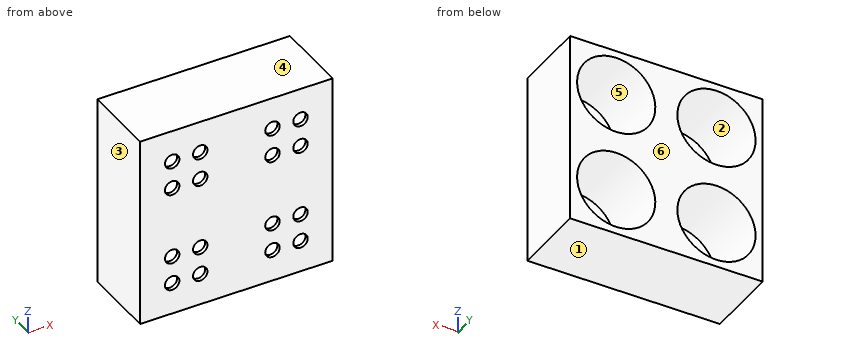
```python
from build123d import *

# Parameters (mm, degrees)
SKETCH1_W           = 96
SKETCH1_H           = 96
SKETCH1_R           = 19.5
BOSS_EXTRUDE1_DEPTH = 35
SKETCH2_W           = 96
SKETCH2_H           = 96
BOSS_EXTRUDE2_DEPTH = 2
SKETCH3_R           = 3.6
CUT_EXTRUDE1_DEPTH  = 110.009173926


with BuildPart() as part:
    # Sketch1 → Boss-Extrude1 (new body)
    with BuildSketch(Plane(origin=(0, 0, 0), x_dir=(1, 0, 0), z_dir=(0, 1, 0))):
        with Locations((25, 25)):
            Rectangle(SKETCH1_W, SKETCH1_H)
        with Locations(Location((0, 0, 0), (0, 0, 270))):
            Circle(SKETCH1_R, mode=Mode.SUBTRACT)
        with Locations(Location((50, 0, 0), (0, 0, 270))):
            Circle(SKETCH1_R, mode=Mode.SUBTRACT)
        with Locations(Location((50, 50, 0), (0, 0, 270))):
            Circle(SKETCH1_R, mode=Mode.SUBTRACT)
        with Locations(Location((0, 50, 0), (0, 0, 270))):
            Circle(SKETCH1_R, mode=Mode.SUBTRACT)
    extrude(amount=BOSS_EXTRUDE1_DEPTH)

    # Sketch2 → Boss-Extrude2 (add)
    with BuildSketch(Plane.XZ):
        with Locations((25, -25)):
            Rectangle(SKETCH2_W, SKETCH2_H)
    extrude(amount=BOSS_EXTRUDE2_DEPTH)

    # Sketch3 → Cut-Extrude1 (cut, through all)
    with BuildSketch(Plane(origin=(0, 0, 0), x_dir=(1, 0, 0), z_dir=(0, 1, 0))):
        with Locations(Location((57, 43, 0), (0, 0, 270))):
            Circle(SKETCH3_R)
        with Locations(Location((57, 57, 0), (0, 0, 90))):
            Circle(SKETCH3_R)
        with Locations(Location((43, 43, 0), (0, 0, 90))):
            Circle(SKETCH3_R)
        with Locations(Location((43, 57, 0), (0, 0, 270))):
            Circle(SKETCH3_R)
        with Locations(Location((57, 7, 0), (0, 0, 270))):
            Circle(SKETCH3_R)
        with Locations(Location((43, 7, 0), (0, 0, 90))):
            Circle(SKETCH3_R)
        with Locations(Location((43, -7, 0), (0, 0, 270))):
            Circle(SKETCH3_R)
        with Locations(Location((57, -7, 0), (0, 0, 90))):
            Circle(SKETCH3_R)
        with Locations(Location((7, 7, 0), (0, 0, 270))):
            Circle(SKETCH3_R)
        with Locations(Location((7, -7, 0), (0, 0, 90))):
            Circle(SKETCH3_R)
        with Locations(Location((-7, -7, 0), (0, 0, 270))):
            Circle(SKETCH3_R)
        with Locations(Location((-7, 7, 0), (0, 0, 90))):
            Circle(SKETCH3_R)
        with Locations(Location((7, 57, 0), (0, 0, 270))):
            Circle(SKETCH3_R)
        with Locations(Location((7, 43, 0), (0, 0, 90))):
            Circle(SKETCH3_R)
        with Locations(Location((-7, 43, 0), (0, 0, 270))):
            Circle(SKETCH3_R)
        with Locations(Location((-7, 57, 0), (0, 0, 90))):
            Circle(SKETCH3_R)
    extrude(amount=-CUT_EXTRUDE1_DEPTH, mode=Mode.SUBTRACT)


solid = part.part
```
CAD build for the part. Positions are in the model's coordinates, mm. Face numbers are marked on the shaded views. A direction names the side the tool comes from. Coordinates: 2 decimals unless noted, no trailing zeros. Write each loop counter-clockwise with the first axis right and the second up, starting at its lowest first coordinate (ties: lowest second). Pieces come first, ordered by that corner, then holes. Notation, with made-up numbers: (-10.75, -3.75) -> (27.25, -3.75) arc R16 ccw to (27.25, 23.25) -> close; hole circle Ø8 at (79, 74). An arc over 180 degrees is marked (long way). Return JSON: item names as keys, results as strings. Group by question number.
Q1. Flat gauge pins, fed straight in: pin 1 (6 mm diameter, centred on x = 7, z = 7, fed in from -Y); pin 2 (11.5 mm diameter, centred on x = 43, z = -7, fed in from +Y). Where does each tip first touch, or does it go through?
Q2. Cut at C-C, the plane z = -43.5. Give the cut face in (x, y).
Q3. Which spindle directions (+Z, -Z, +X, -X, +Y, -Y) get a long thin tool onto all of the face, cutting with end or side? Do the marked faces 5 and 6. Say none if no direction does.
Q4. Cut at A-A, the plane y = 10. Give the cut face in (x, z).
Q5. Cut at B-B, the plane x = 0. Give the cut face in (y, z).
Q6. Pull direction Z, two halves, no side cores. Call the marked faces 1, 2, 3 and 4: released by +Z, released by -Z, zero draft, split by the parting line, or undercut.
Q7. Drill centre lines: line 1 (X direction, y = -1.15, z = -43); line 2 (Z direction, x = 39, y = 29); line 3 (Z direction, x = 57, y = 21.5). Where is each one in solid material? Low to high.
Q8. Cut at D-D, the plane z = 0. Give the cut face in (x, y), then the cut area to 3 significant figures.
Returned:
{
 "1": {"pin 1": "passes through", "pin 2": "stops at y = 0"},
 "2": {"outline": "(-23, -2) -> (-10.57, -2) -> (-10.57, 0) -> (-18.38, 0) -> (-18.38, 35) -> (-23, 35) -> close; (-3.43, -2) -> (3.43, -2) -> (3.43, 0) -> (-3.43, 0) -> close; (10.57, -2) -> (39.43, -2) -> (39.43, 0) -> (31.62, 0) -> (31.62, 35) -> (18.38, 35) -> (18.38, 0) -> (10.57, 0) -> close; (46.57, -2) -> (53.43, -2) -> (53.43, 0) -> (46.57, 0) -> close; (60.57, -2) -> (73, -2) -> (73, 35) -> (68.38, 35) -> (68.38, 0) -> (60.57, 0) -> close"},
 "3": {"face 5": "+Y", "face 6": "+Z, -Z, +X, -X, +Y"},
 "4": {"outline": "(-23, -73) -> (73, -73) -> (73, 23) -> (-23, 23) -> close; hole circle Ø39 at (0, -50); hole circle Ø39 at (0, 0); hole circle Ø39 at (50, -50); hole circle Ø39 at (50, 0)"},
 "5": {"outline": "(-2, -73) -> (35, -73) -> (35, -69.5) -> (0, -69.5) -> (0, -30.5) -> (35, -30.5) -> (35, -19.5) -> (0, -19.5) -> (0, 19.5) -> (35, 19.5) -> (35, 23) -> (-2, 23) -> close"},
 "6": {"face 1": "released by -Z", "face 2": "undercut", "face 3": "zero draft", "face 4": "released by +Z"},
 "7": {"line 1": "x = -23 to -10.6, -3.4 to 3.4, 10.6 to 39.4, 46.6 to 53.4, 60.6 to 73", "line 2": "z = -73 to -66.1, -33.9 to -16.1, 16.1 to 23", "line 3": "z = -73 to -68.2, -31.8 to -18.2, 18.2 to 23"},
 "8": {"outline": "(-23, -2) -> (73, -2) -> (73, 35) -> (69.5, 35) -> (69.5, 0) -> (30.5, 0) -> (30.5, 35) -> (19.5, 35) -> (19.5, 0) -> (-19.5, 0) -> (-19.5, 35) -> (-23, 35) -> close", "area": "822 mm2"}
}
